The drawing under review shows one solid part. Ordinate dimensions are in mm from its lowest x, y, z. Give positions to 0.01 mm unless a question says otherwise; leave off trailing zeros. Loops run counter-clockwise (first coordinate to the right, second up) from the corner with the lowest first, then second, coordinate; pieces in that order, holes last. Notation, with made-up numbers: (-38, 9) -> (2, 9) arc R10 cw to (2, 21) -> close; hole circle Ø10 at (85, 6). An arc over 180 degrees is marked (long way). Answer in a Markdown table with one row per item. Add a question column.
(1) Consider section C-C on x = 5. Write out the cut boundary in (y, z).
(2) Consider section A-A on y = 6. Write out the cut boundary in (x, z), then the cut area to 3 significant figures.
(3) Consider section B-B on x = 100. Write out the cut boundary in (y, z).
(4) For pin 1 (3.5 mm diameter, centred on x = 40, y = 6, fed in from +Z), flat-tipped, find the tip position at first contact; note if it passes through.
(5) For line 1 (Y direction, x = 100, z = 1.5); line 2 (Y direction, x = 195, z = 2.5); line 3 (X direction, y = 52.5, z = 6), list the stretches that pass through material, from the lowest coordinate up.
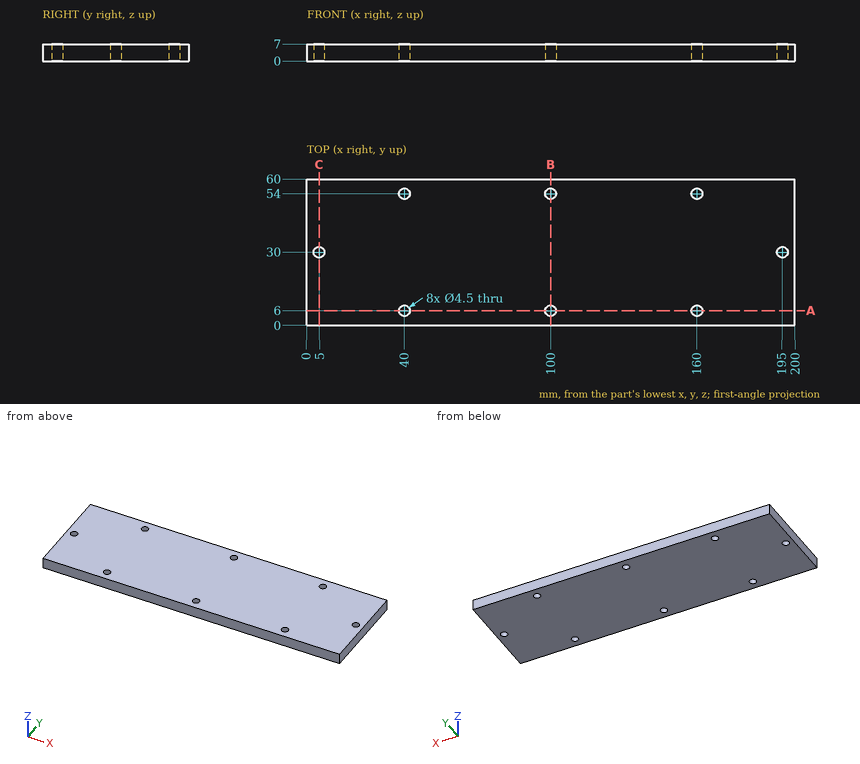
Values follow:
| question | item | result |
|---|---|---|
| 1 | outline | (0, 0) -> (27.75, 0) -> (27.75, 7) -> (0, 7) -> close; (32.25, 0) -> (60, 0) -> (60, 7) -> (32.25, 7) -> close |
| 2 | outline | (0, 0) -> (37.75, 0) -> (37.75, 7) -> (0, 7) -> close; (42.25, 0) -> (97.75, 0) -> (97.75, 7) -> (42.25, 7) -> close; (102.25, 0) -> (157.75, 0) -> (157.75, 7) -> (102.25, 7) -> close; (162.25, 0) -> (200, 0) -> (200, 7) -> (162.25, 7) -> close |
| 2 | area | 1,310 mm2 |
| 3 | outline | (0, 0) -> (3.75, 0) -> (3.75, 7) -> (0, 7) -> close; (8.25, 0) -> (51.75, 0) -> (51.75, 7) -> (8.25, 7) -> close; (56.25, 0) -> (60, 0) -> (60, 7) -> (56.25, 7) -> close |
| 4 | pin 1 | through |
| 5 | line 1 | 0 to 3.75, 8.25 to 51.75, 56.25 to 60 |
| 5 | line 2 | 0 to 27.75, 32.25 to 60 |
| 5 | line 3 | 0 to 38.32, 41.68 to 98.32, 101.68 to 158.32, 161.68 to 200 |
